Design review of the part built by this model. Coordinates are the model's own, in mm. A direction names the side the tool comes from. Coordinates: 2 decimals unless noted, no trailing zeros. Write each loop counter-clockwise with the first axis right and the second up, starting at its lowest first coordinate (ties: lowest second). Pieces come first, ordered by that corner, then holes.
Q1. Take a section at B-B, the plane y = -161. Write out the cut boundary in (x, z).
Q2. Take a section at C-C, the plane x = -30. Write out the cut boundary in (y, z), plus the area to 3 significant figures.
Q3. For pin 1 Ø6 at (y, z) = (-77, 63) entering from -X; pin 2 Ø7.5 at (x, z) = (23, 68.5) entering from +Y; pin 3 Ø7.5 at (y, z) = (-108, 65.5) entering from +X, all flat-tipped, find the tip position at first contact; note any pin that passes through.
Q4. Take a section at D-D, the plane y = -78.5. Write out the cut boundary in (x, z), plus the area to 3 significant figures.
Q5. For L1, parallel to X at y = -161, z = 63; L2, parallel to Y at x = -30, z = 71; L3, parallel to Z at x = 2, y = 0, list the stretches that pass through material, from the lowest coordinate up.
Q6. The part is to be moulded in two halves that separate along X. For faces 1 (the cylindrical face through (4.289, 4.196, 66.605)), 2 (the flat face through (-1, 0, 0)), 3 (the cylindrical face through (-30, -158, 67)), say which applies: released by +X, released by -X, zero draft, split by the parting line, or undercut.
Q7. Take a section at A-A, the plane z = 66.5. State how many separate pieces and enclosed holes the cut face has, plus the area to 3 significant figures.
Q8. For faces 4 (the cylindrical face through (0.084, 0.751, 64.115)), 5 (the flat face through (-20, -156, 67)), 6 (the flat face through (21, -156, 67)), 7 (the flat face through (2, -2, 29)), 8 (the flat face through (0, -166, 67)), list the 3-axis set-ups (+Z, -Z, +X, -X, +Y, -Y) from which the entire face can be reached by the end or side of a thin tool; tool diameter is ignored.
from build123d import *

# Parameters (mm, degrees)
BOSS_EXTRU_1_DEPTH      = 59
BOSS_EXTRU_2_DEPTH      = 15
CONG_1_R                = 6
BOSS_EXTRU_3_DEPTH      = 150
ESQUISSE5_W             = 15
ESQUISSE5_H             = 10
BOSS_EXTRU_4_DEPTH      = 35
ENL_V_MAT_EXTRU_1_REACH = 187.086
ESQUISSE6_R             = 3
ENL_V_MAT_EXTRU_2_REACH = 188.314


with BuildPart() as part:
    # Esquisse1 → Boss.-Extru.1 (new body)
    with BuildSketch(Plane.XY):
        with BuildLine():
            Line((4.242640687, -4.242640687), (0, 0))
            Line((0, 0), (0, 6))
            ThreePointArc((0, 6), (-5.543277195, -2.296100594), (4.242640687, -4.242640687))
        make_face()
        with BuildLine():
            Line((0, 6), (0, 0))
            Line((0, 0), (4.242640687, 4.242640687))
            ThreePointArc((4.242640687, 4.242640687), (2.296100594, 5.543277195), (0, 6))
        make_face()
    extrude(amount=BOSS_EXTRU_1_DEPTH)

    # Esquisse2 → Boss.-Extru.2 (add)
    with BuildSketch(Plane.XY.offset(59)):
        with BuildLine():
            ThreePointArc((0, -6), (-4.242640708, -4.242640666), (-6, 5.9e-08))
            Line((-6, 5.9e-08), (-6, -6))
            Line((-6, -6), (0, -6))
        make_face()
        with BuildLine():
            Line((0, 0), (0, 6))
            ThreePointArc((0, 6), (-4.242640666, 4.242640708), (-6, 5.9e-08))
            ThreePointArc((-6, 5.9e-08), (-4.242640708, -4.242640666), (0, -6))
            Line((0, -6), (0, 0))
        make_face()
        with BuildLine():
            ThreePointArc((4.242640687, 4.242640687), (2.296100594, 5.543277195), (0, 6))
            Line((0, 6), (0, 0))
            Line((0, 0), (4.242640687, 4.242640687))
        make_face()
        with BuildLine():
            Line((6, 6), (0, 6))
            ThreePointArc((0, 6), (2.296100594, 5.543277195), (4.242640687, 4.242640687))
            Line((4.242640687, 4.242640687), (0, 0))
            Line((0, 0), (4.242640687, -4.242640687))
            ThreePointArc((4.242640687, -4.242640687), (2.296100594, -5.543277195), (0, -6))
            Line((0, -6), (6, -6))
            Line((6, -6), (6, 6))
        make_face()
        with BuildLine():
            ThreePointArc((-6, 5.9e-08), (-4.242640666, 4.242640708), (0, 6))
            Line((0, 6), (-6, 6))
            Line((-6, 6), (-6, 5.9e-08))
        make_face()
        with BuildLine():
            Line((4.242640687, -4.242640687), (0, 0))
            Line((0, 0), (0, -6))
            ThreePointArc((0, -6), (2.296100594, -5.543277195), (4.242640687, -4.242640687))
        make_face()
    extrude(amount=BOSS_EXTRU_2_DEPTH)

    # Congé1
    cong_1_edges = [part.edges().sort_by_distance(p)[0] for p in [
        (6, 6, 66.5),
        (-6, 6, 66.5),
    ]]
    fillet(cong_1_edges, radius=CONG_1_R - 0.0001)  # a hair under: the kernel refuses the full size

    # Esquisse4 → Boss.-Extru.3 (add)
    with BuildSketch(Plane.XZ.offset(6)):
        Polygon((0, 59), (6, 59), (6, 74), (-6, 74), (-6, 59), align=None)
    extrude(amount=BOSS_EXTRU_3_DEPTH)

    # Esquisse5 → Boss.-Extru.4 (add, symmetric)
    with BuildSketch(Plane(origin=(0, 0, 0), x_dir=(0, 0, -1), z_dir=(1, 0, 0))):
        with Locations((-66.5, -161)):
            Rectangle(ESQUISSE5_W, ESQUISSE5_H)
    extrude(amount=BOSS_EXTRU_4_DEPTH, both=True)

    # Esquisse6 → Enlèv. mat.-Extru.1 (cut, up to next)
    with BuildSketch(Plane.XY.offset(74), mode=Mode.PRIVATE) as enl_v_mat_extru_1_sk1:
        with Locations((-30, -161)):
            Circle(ESQUISSE6_R)
    enl_v_mat_extru_1_tool1 = extrude(enl_v_mat_extru_1_sk1.sketch, amount=-ENL_V_MAT_EXTRU_1_REACH, mode=Mode.PRIVATE) & part.part
    # Esquisse6 → Enlèv. mat.-Extru.1 (cut, up to next)
    with BuildSketch(Plane.XY.offset(74), mode=Mode.PRIVATE) as enl_v_mat_extru_1_sk2:
        with Locations((30, -161)):
            Circle(ESQUISSE6_R)
    enl_v_mat_extru_1_tool2 = extrude(enl_v_mat_extru_1_sk2.sketch, amount=-ENL_V_MAT_EXTRU_1_REACH, mode=Mode.PRIVATE) & part.part
    add(enl_v_mat_extru_1_tool1.solids().sort_by_distance((-30, -161, 74))[0], mode=Mode.SUBTRACT)
    add(enl_v_mat_extru_1_tool2.solids().sort_by_distance((30, -161, 74))[0], mode=Mode.SUBTRACT)

    # Esquisse7 → Enlèv. mat.-Extru.2 (cut, up to next)
    with BuildSketch(Plane(origin=(6, 0, 0), x_dir=(0, 0, -1), z_dir=(1, 0, 0)), mode=Mode.PRIVATE) as enl_v_mat_extru_2_sk1:
        with BuildLine():
            ThreePointArc((-69, 0), (-66.5, -2.5), (-64, 0))
            Line((-64, 0), (-69, 0))
        make_face()
    enl_v_mat_extru_2_tool1 = extrude(enl_v_mat_extru_2_sk1.sketch, amount=-ENL_V_MAT_EXTRU_2_REACH, mode=Mode.PRIVATE) & part.part
    # Esquisse7 → Enlèv. mat.-Extru.2 (cut, up to next)
    with BuildSketch(Plane(origin=(6, 0, 0), x_dir=(0, 0, -1), z_dir=(1, 0, 0)), mode=Mode.PRIVATE) as enl_v_mat_extru_2_sk2:
        with BuildLine():
            Line((-69, 0), (-64, 0))
            ThreePointArc((-64, 0), (-66.5, 2.5), (-69, 0))
        make_face()
    enl_v_mat_extru_2_tool2 = extrude(enl_v_mat_extru_2_sk2.sketch, amount=-ENL_V_MAT_EXTRU_2_REACH, mode=Mode.PRIVATE) & part.part
    # Esquisse7 → Enlèv. mat.-Extru.2 (cut, up to next)
    with BuildSketch(Plane(origin=(6, 0, 0), x_dir=(0, 0, -1), z_dir=(1, 0, 0)), mode=Mode.PRIVATE) as enl_v_mat_extru_2_sk3:
        with BuildLine():
            ThreePointArc((-69, 0), (-66.5, -2.5), (-64, 0))
            Line((-64, 0), (-69, 0))
        make_face()
    enl_v_mat_extru_2_tool3 = extrude(enl_v_mat_extru_2_sk3.sketch, amount=-ENL_V_MAT_EXTRU_2_REACH, mode=Mode.PRIVATE) & part.part
    # Esquisse7 → Enlèv. mat.-Extru.2 (cut, up to next)
    with BuildSketch(Plane(origin=(6, 0, 0), x_dir=(0, 0, -1), z_dir=(1, 0, 0)), mode=Mode.PRIVATE) as enl_v_mat_extru_2_sk4:
        with BuildLine():
            Line((-69, 0), (-64, 0))
            ThreePointArc((-64, 0), (-66.5, 2.5), (-69, 0))
        make_face()
    enl_v_mat_extru_2_tool4 = extrude(enl_v_mat_extru_2_sk4.sketch, amount=-ENL_V_MAT_EXTRU_2_REACH, mode=Mode.PRIVATE) & part.part
    add(enl_v_mat_extru_2_tool1.solids().sort_by_distance((6, -1.061033, 66.5))[0], mode=Mode.SUBTRACT)
    add(enl_v_mat_extru_2_tool2.solids().sort_by_distance((6, 1.061033, 66.5))[0], mode=Mode.SUBTRACT)
    add(enl_v_mat_extru_2_tool3.solids().sort_by_distance((6, -1.061033, 66.5))[0], mode=Mode.SUBTRACT)
    add(enl_v_mat_extru_2_tool4.solids().sort_by_distance((6, 1.061033, 66.5))[0], mode=Mode.SUBTRACT)


solid = part.part
Responses:
1. outline: (-35, 59) - (-33, 59) - (-33, 74) - (-35, 74) - close; (-27, 59) - (27, 59) - (27, 74) - (-27, 74) - close; (33, 59) - (35, 59) - (35, 74) - (33, 74) - close
2. outline: (-166, 59) - (-164, 59) - (-164, 74) - (-166, 74) - close; (-158, 59) - (-156, 59) - (-156, 74) - (-158, 74) - close
2. area: 60.0 mm2
3. pin 1: stops at x = -6
3. pin 2: stops at y = -156
3. pin 3: stops at x = 6
4. outline: (-6, 59) - (6, 59) - (6, 74) - (-6, 74) - close
4. area: 180 mm2
5. L1: x = -35 to -33, -27 to 27, 33 to 35
5. L2: y = -166 to -164, -158 to -156
5. L3: z = 59 to 64, 69 to 74
6. face 1: released by +X
6. face 2: zero draft
6. face 3: undercut
7. separate pieces: 2
7. enclosed holes: 2
7. area: 2,510 mm2
8. face 4: +X, -X
8. face 5: +Z, -Z, -X, +Y
8. face 6: +Z, -Z, +X, +Y
8. face 7: -Z, +X
8. face 8: +Z, -Z, +X, -X, -Y
